from build123d import *

# Parameters (mm, degrees)
SKETCH1_W           = 316.8
SKETCH1_H           = 457.2
BOSS_EXTRUDE1_DEPTH = 6
SKETCH2_R           = 37
CUT_EXTRUDE1_DEPTH  = 279.180732618
SKETCH3_W           = 316.8
SKETCH3_H           = 146.4
CUT_EXTRUDE2_DEPTH  = 279.180732618
SKETCH4_R           = 3
CUT_EXTRUDE3_DEPTH  = 279.180732618


with BuildPart() as part:
    # Sketch1 → Boss-Extrude1 (new body)
    with BuildSketch(Plane.XY):
        Rectangle(SKETCH1_W, SKETCH1_H)
    extrude(amount=BOSS_EXTRUDE1_DEPTH)

    # Sketch2 → Cut-Extrude1 (cut, through all)
    with BuildSketch(Plane.XY.offset(6)):
        with Locations((0, 173.6)):
            Circle(SKETCH2_R)
    extrude(amount=-CUT_EXTRUDE1_DEPTH, mode=Mode.SUBTRACT)

    # Sketch3 → Cut-Extrude2 (cut, through all)
    with BuildSketch(Plane.XY.offset(6)):
        with Locations((0, -155.4)):
            Rectangle(SKETCH3_W, SKETCH3_H)
    extrude(amount=-CUT_EXTRUDE2_DEPTH, mode=Mode.SUBTRACT)

    # Sketch4 → Cut-Extrude3 (cut, through all)
    with BuildSketch(Plane.XY.offset(6)):
        with Locations((-133.4, 203.6)):
            Circle(SKETCH4_R)
        with Locations((-133.4, -57.2)):
            Circle(SKETCH4_R)
        with Locations((133.4, -57.2)):
            Circle(SKETCH4_R)
        with Locations((133.4, 203.6)):
            Circle(SKETCH4_R)
    extrude(amount=-CUT_EXTRUDE3_DEPTH, mode=Mode.SUBTRACT)


solid = part.part
Can you work these out from the model? Positions are in its coordinate system, mm. Round coordinates to 2 decimals unless told otherwise and drop trailing zeros. Write each loop counter-clockwise with the first axis right and the second up, starting at its lowest first coordinate (ties: lowest second). Pieces come first, ordered by that corner, then holes. Notation, with made-up numbers: (-33, 21) - (-11, 21) arc R20 ccw to (-11, 40) - close; hole circle Ø8 at (32, 84). An arc over 180 degrees is marked (long way). Write each question's results on one line, items separated by ' | '. Start each with the question number.
1) Suppose I cut it at B-B (x = 0). List the corners of the cut face in (y, z) for me.
2) We'd pull the mould along X, two halves only. Please class faces 1 (the flat face through (-2, 75, 6)), 2 (the cylindrical face through (-4.817, 210.285, 3.042)): released by +X, released by -X, zero draft, split by the parting line, or undercut.
3) For pin 1 Ø5 at (x, y) = (133.4, 203.6) entering from -Z, with a flat end and sliding along its axis, tell me the tip position at first contact or that it passes through.
4) Please list where these lines run through material, in increasing order: line 1 (Y direction, x = 133.4, z = 2.6); line 2 (Y direction, x = 0, z = 3.45); line 3 (X direction, y = 189, z = 3.35).
5) Suppose I cut it at C-C (z = 3.4). List the corners of the cut face in (x, y) for me, and give its area (3 significant figures).
6) Suppose I cut it at A-A (y = 173.6). List the corners of the cut face in (x, z) for me.
Here are the results:
1) outline: (-82.2, 0) - (136.6, 0) - (136.6, 6) - (-82.2, 6) - close; (210.6, 0) - (228.6, 0) - (228.6, 6) - (210.6, 6) - close
2) face 1: zero draft | face 2: undercut
3) pin 1: passes through
4) line 1: y = -82.2 to -60.2, -54.2 to 200.6, 206.6 to 228.6 | line 2: y = -82.2 to 136.6, 210.6 to 228.6 | line 3: x = -158.4 to -33.64, 33.64 to 158.4
5) outline: (-158.4, -82.2) - (158.4, -82.2) - (158.4, 228.6) - (-158.4, 228.6) - close; hole circle Ø6 at (-133.4, -57.2); hole circle Ø6 at (-133.4, 203.6); hole circle Ø74 at (0, 173.6); hole circle Ø6 at (133.4, -57.2); hole circle Ø6 at (133.4, 203.6) | area: 94,000 mm2
6) outline: (-158.4, 0) - (-37, 0) - (-37, 6) - (-158.4, 6) - close; (37, 0) - (158.4, 0) - (158.4, 6) - (37, 6) - close
